Solid Edge part; units mm, degrees
sketch "Sketch1" plane through (0, 0, 0) normal (0, 0, 1) x (1, 0, 0)
  arc A0 (-12, 0) -> (6.6023, 10.0204) centre (0, 0) cw
  line L0 (6.6023, 10.0204) -> (12, 6.464)
  line L1 (12, 6.464) -> (31.356, 6.464)
  line L2 (31.356, 6.464) -> (31.356, 8)
  line L3 (31.356, 8) -> (36, 8)
  line L4 (36, 8) -> (36, 0)
  line L5 (36, 0) -> (-12, 0)
revolve "RevolvedProtrusion1" add sketch "Sketch1" angle 360 about axis through (36, 0, 0) along (-1, 0, 0)
sketch "Sketch2" plane through (0, 0, 0) normal (0, 0, 1) x (1, 0, 0)
  line L0 (-16, -12.1) -> (25.1636, -12.1)
  line L1 (25.1636, -12.1) -> (12, -4.5)
  line L2 (12, -4.5) -> (-15, -4.5)
  line L3 (-15, -4.5) -> (-15, 4.5)
  line L4 (-15, 4.5) -> (12, 4.5)
  line L5 (12, 4.5) -> (25.1636, 12.1)
  line L6 (25.1636, 12.1) -> (-16, 12.1)
  line L7 (-16, 12.1) -> (-16, -12.1)
extrude "ExtrudedCutout_1" cut sketch "Sketch2" against normal blind 12 and the other way blind 12
sketch "Sketch3" plane through (36, 0, 0) normal (1, 0, 0) x (0, 1, 0)
  line L0 (-14, -14) -> (-7, -14)
  line L1 (-7, -14) -> (-7, 12)
  line L2 (-7, 12) -> (7, 12)
  line L3 (7, 12) -> (7, -14)
  line L4 (7, -14) -> (14, -14)
  line L5 (14, -14) -> (14, 14)
  line L6 (14, 14) -> (-14, 14)
  line L7 (-14, 14) -> (-14, -14)
extrude "ExtrudedCutout_2" cut sketch "Sketch3" against normal blind 16 and the other way blind 16
sketch "Sketch4" plane through (0, 0, 0) normal (0, 0, 1) x (1, 0, 0)
  line L0 (14.0812, 0) -> (16, 3.3235)
  line L1 (16, 3.3235) -> (35.3235, 3.3235)
  line L2 (35.3235, 3.3235) -> (36, 4)
  line L3 (36, 4) -> (36, 0)
  line L4 (36, 0) -> (14.0812, 0)
revolve "RevolvedCutout1" cut sketch "Sketch4" angle 360 about axis through (36, 0, 0) along (-1, 0, 0)
cosmetic_thread "Thread_1" thread depth 14.323
sketch "Sketch5" plane through (0, 0, 0) normal (0, 0, 1) x (1, 0, 0)
  line L0 (0, 6) -> (5.9699, 6)
  arc A0 (5.9699, 6) -> (5.9699, -6) centre (0, 0) cw
  line L1 (5.9699, -6) -> (0, -6)
  line L2 (0, -6) -> (0, 6)
revolve "RevolvedProtrusion2" add sketch "Sketch5" angle 360 about axis through (0, -6, 0) along (0, 1, 0)
sketch "Sketch6" plane through (0, 0, 0) normal (0, 0, 1) x (1, 0, 0)
  line L0 (0, 8) -> (4, 8)
  line L1 (4, 8) -> (4, -8)
  line L2 (4, -8) -> (0, -8)
  line L3 (0, -8) -> (0, 8)
revolve "RevolvedCutout2" cut sketch "Sketch6" angle 360 about axis through (0, -8, 0) along (0, 1, 0)
properties part number "195581 CRSGS-M8---(K_0)"
Source: CAD feature listing. Evaluate the final solid. Frame: model axes, mm. A direction names the side the tool comes from. Give positions to 0.01 mm unless a question says otherwise; leave off trailing zeros. Order: outer loops, then holes, each group sorted by start corner. A loop starts at its lowest first (then second) coordinate and runs counter-clockwise, first axis right, second up. Notation, with made-up numbers: (-13, -30.75) -> (31, -30.75) arc R28 ccw to (31, -5.75) -> close; hole circle Ø10 at (-33.5, -10). An arc over 180 degrees is marked (long way). Use a Markdown table: item, result.
Q1. Pull-direction query (Y, two-part tool) for faces 1 (the face through (25.8, 3.07, -1.27)), 2 (the face through (9.863, -0.085, 7.871)), 3 (the face through (34, -7, 0)); classes: +Y half, -Y half, draft (parallel to the pull), parting line (faces both ways), or undercut.
A:
| item | result |
|---|---|
| face 1 | undercut |
| face 2 | parting line |
| face 3 | -Y half |
Q2. First-contact query: P1, Ø1, axis at y = -1.5, z = 7.5, coming from the -X side; P2, Ø12, axis at x = 2, z = 5.5, coming from the +Y side; P3, Ø1.5, axis at x = 10.5, z = -1.5, coming from the +Y side. Flat tips, straight axial feed; report the tip coordinate or a pass-through.
A:
| item | result |
|---|---|
| P1 | x = -9.64 |
| P2 | y = 6 |
| P3 | y = 4.5 |
Q3. Access query for faces 4 (the face through (34, 0, 8)), 5 (the face through (13.35, -5.28, 0.06)), 6 (the face through (34, 0, -8)), 7 (the face through (9.863, 0.085, -7.871)). Directions: +Z, -Z, +X, -X, +Y, -Y. A direction counts if a zero-diameter tool reaches every point of the face in a straight line with its end or side. Return the directions, or none.
A:
| item | result |
|---|---|
| face 4 | +Z, +X |
| face 5 | +Z, -Z, -Y |
| face 6 | -Z, +X |
| face 7 | -Z |
Q4. Section B-B (y = -5.25). Return the cut outline in (x, z).
A:
| item | result |
|---|---|
| outline | circle Ø13.28 at (0, 0); (13.3, -3.77) -> (31.36, -3.77) -> (31.36, -6.04) -> (36, -6.04) -> (36, 6.04) -> (31.36, 6.04) -> (31.36, 3.77) -> (13.3, 3.77) -> close; hole circle Ø8 at (0, 0) |
Q5. Section A-A (x = 0). Return the cut outline in (y, z).
A:
| item | result |
|---|---|
| outline | (-6, -5.97) arc R8.46 ccw to (-4.5, -7.17) -> (-4.5, -11.12) arc R12 ccw to (4.5, -11.12) -> (4.5, -7.17) arc R8.46 ccw to (6, -5.97) -> (6, -4) -> (-6, -4) -> close; (-6, 4) -> (6, 4) -> (6, 5.97) arc R8.46 ccw to (4.5, 7.17) -> (4.5, 11.12) arc R12 ccw to (-4.5, 11.12) -> (-4.5, 7.17) arc R8.46 ccw to (-6, 5.97) -> close |
Q6. Material intervals for line 1 (X direction, y = 5.25, z = 0.75); line 2 (Y direction, x = 27.5, z = 0); line 3 (Z direction, x = 24, y = 0.25), sorted ascending. Write a range as [from, to].
A:
| item | result |
|---|---|
| line 1 | [-6.6, -3.93], [3.93, 6.6], [13.3, 36] |
| line 2 | [-6.46, -3.32], [3.32, 6.46] |
| line 3 | [-6.46, -3.31], [3.31, 6.46] |
Q7. Section C-C (x = 29.5). Return the cut outline in (y, z).
A:
| item | result |
|---|---|
| outline | circle Ø12.93 at (0, 0); hole circle Ø6.65 at (0, 0) |
